```python
from build123d import *

# Parameters (mm, degrees)
SKETCH1_R           = 1.75
BOSS_EXTRUDE1_DEPTH = 4
SKETCH2_W           = 8
SKETCH2_H           = 88.5
BOSS_EXTRUDE2_DEPTH = 5
FILLET1_R           = 2
SKETCH3_R           = 1.75
CUT_EXTRUDE1_DEPTH  = 145.395290782


with BuildPart() as part:
    # Sketch1 → Boss-Extrude1 (new body)
    with BuildSketch(Plane.XY):
        with BuildLine():
            Line((-26.5, 140), (-35, 140))
            Line((-35, 140), (-35, 0))
            Line((-35, 0), (35, 0))
            Line((35, 0), (35, 140))
            Line((35, 140), (26.5, 140))
            ThreePointArc((26.5, 140), (0, 113.5), (-26.5, 140))
        make_face()
        with Locations((-25, 60)):
            Circle(SKETCH1_R, mode=Mode.SUBTRACT)
        with Locations((25, 60)):
            Circle(SKETCH1_R, mode=Mode.SUBTRACT)
        with Locations((-10, 10)):
            Circle(SKETCH1_R, mode=Mode.SUBTRACT)
        with Locations((10, 10)):
            Circle(SKETCH1_R, mode=Mode.SUBTRACT)
        with Locations((10, 20)):
            Circle(SKETCH1_R, mode=Mode.SUBTRACT)
        with Locations((-10, 20)):
            Circle(SKETCH1_R, mode=Mode.SUBTRACT)
        with Locations((10, 30)):
            Circle(SKETCH1_R, mode=Mode.SUBTRACT)
        with Locations((-10, 30)):
            Circle(SKETCH1_R, mode=Mode.SUBTRACT)
    extrude(amount=BOSS_EXTRUDE1_DEPTH)

    # Sketch2 → Boss-Extrude2 (add)
    with BuildSketch(Plane.XY.offset(4)):
        with Locations((0, 65.75)):
            Rectangle(SKETCH2_W, SKETCH2_H)
    extrude(amount=BOSS_EXTRUDE2_DEPTH)

    # Fillet1
    fillet1_edges = [part.edges().sort_by_distance(p)[0] for p in [
        (-4, 65.75, 9),
        (4, 65.75, 9),
    ]]
    fillet(fillet1_edges, radius=FILLET1_R)

    # Sketch3 → Cut-Extrude1 (cut, through all)
    with BuildSketch(Plane.XY.offset(4)):
        with Locations((-25, 90)):
            Circle(SKETCH3_R)
        with Locations((25, 90)):
            Circle(SKETCH3_R)
    extrude(amount=-CUT_EXTRUDE1_DEPTH, mode=Mode.SUBTRACT)


solid = part.part
```
Could you check a few things on this model? Use its own coordinates, in mm. A direction names the side the tool comes from. Give positions to 0.01 mm unless a question says otherwise; leave off trailing zeros. Loops run counter-clockwise (first coordinate to the right, second up) from the corner with the lowest first, then second, coordinate; pieces in that order, holes last. Notation, with made-up numbers: (0, 25.25) - (24, 25.25) arc R30 cw to (24, 47.25) - close; hole circle Ø3 at (84.25, -21.5). An arc over 180 degrees is marked (long way). Answer in a Markdown table with one row per item. Add a question column.
Q1. We'd pull the mould along Y, two halves only. Please class faces 4 (the face through (-8.331, 30.526, 1.972)), 5 (the face through (35, 69, 2)), 6 (the face through (31, 140, 2)), 7 (the face through (9.772, 21.735, 1.972)): +Y half, -Y half, draft (parallel to the pull), parting line (faces both ways), or undercut.
Q2. If we section it at A-A (y = 10): List the corners of the cut face in (x, z) for me, plus the area to 3 significant figures.
Q3. If we section it at B-B (x = 10): List the corners of the cut face in (y, z) for me, plus the area to 3 significant figures.
Q4. If we section it at D-D (x = 25): List the corners of the cut face in (y, z) for me, plus the area to 3 significant figures.
Q5. For pin 1 (21 mm diameter, centred on x = 7.5, y = 58.5, fed in from +Z); pin 2 (4.5 mm diameter, centred on x = 10, y = 10, fed in from +Z); pin 3 (4 mm diameter, centred on x = -26, z = 6.5, fed in from -Y); pin 4 (1.5 mm diameter, centred on x = -1.5, z = 7.5, fed in from -Y), each with a flat end and sliding along its axis, tell me the tip position at first contact or that it passes through.
Q6. Which directions (+Z, -Z, +X, -X, +Y, -Y) give clear straight access to the entire face, cutting with the end or side of a thin tool? Please do faces 1 (the face through (4, 65, 5)), 2 (the face through (0, 21.5, 6)), 3 (the face through (0, 110, 6)).
Q7. Please list where these lines run through material, in increasing order: L1, parallel to Y at x = -10, z = 2.85; L2, parallel to Z at x = 3, y = 18; L3, parallel to Y at x = 0, z = 0.75. Write a range as from..to.
Q8. If we section it at C-C (z = 2): State how many separate pieces and enclosed holes the cut face has, plus the area to 3 significant figures.
The answers:
| question | item | result |
|---|---|---|
| 1 | face 4 | undercut |
| 1 | face 5 | draft |
| 1 | face 6 | +Y half |
| 1 | face 7 | undercut |
| 2 | outline | (-35, 0) - (-11.75, 0) - (-11.75, 4) - (-35, 4) - close; (-8.25, 0) - (8.25, 0) - (8.25, 4) - (-8.25, 4) - close; (11.75, 0) - (35, 0) - (35, 4) - (11.75, 4) - close |
| 2 | area | 252 mm^2 |
| 3 | outline | (0, 0) - (8.25, 0) - (8.25, 4) - (0, 4) - close; (11.75, 0) - (18.25, 0) - (18.25, 4) - (11.75, 4) - close; (21.75, 0) - (28.25, 0) - (28.25, 4) - (21.75, 4) - close; (31.75, 0) - (115.46, 0) - (115.46, 4) - (31.75, 4) - close |
| 3 | area | 420 mm^2 |
| 4 | outline | (0, 0) - (58.25, 0) - (58.25, 4) - (0, 4) - close; (61.75, 0) - (88.25, 0) - (88.25, 4) - (61.75, 4) - close; (91.75, 0) - (131.21, 0) - (131.21, 4) - (91.75, 4) - close |
| 4 | area | 497 mm^2 |
| 5 | pin 1 | stops at z = 9 |
| 5 | pin 2 | stops at z = 4 |
| 5 | pin 3 | passes through |
| 5 | pin 4 | stops at y = 21.5 |
| 6 | face 1 | +Z, +X, +Y, -Y |
| 6 | face 2 | +Z, +X, -X, -Y |
| 6 | face 3 | +Z, +X, -X, +Y |
| 7 | L1 | y = 0..8.25, 11.75..18.25, 21.75..28.25, 31.75..115.46 |
| 7 | L2 | z = 0..4 |
| 7 | L3 | y = 0..113.5 |
| 8 | separate pieces | 1 |
| 8 | enclosed holes | 10 |
| 8 | area | 8,600 mm^2 |
